Autodesk Inventor part; units mm, degrees
ref_plane "YZ Plane" through (0, 0, 0) normal (1, 0, 0) x (0, 1, 0)
ref_plane "XZ Plane" through (0, 0, 0) normal (0, 1, 0) x (-1, 0, 0)
ref_plane "XY Plane" through (0, 0, 0) normal (0, 0, 1) x (1, 0, 0)
sketch "Sketch1" plane through (0, 0, 0) normal (0, 0, 1) x (1, 0, 0)
  line L0 (0, 20.7) -> (0, 15)
  line L1 (29, 15) -> (95, 15)
  line L2 (95, 15) -> (95, 0)
  line L3 (95, 0) -> (-0.5001, 0)
  line L4 (-10.0501, 0) -> (123.65, 0)
  line L5 (-0.5001, 0) -> (-0.5001, 20.7)
  line L6 (-0.5001, 20.7) -> (0, 20.7)
  line L7 (29, 15) -> (26.8528, 15)
  line L8 (26.8528, 15) -> (0, 15)
  line L9 (0, -2.07) -> (0, 26.91)
  dimension "d0" = 95
  dimension "d1" = 66
  dimension "d2" = 30
  dimension "d9" = 0.5001
  dimension "d10" = 41.4
  dimension "d13" = 2.1472
  dimension "d14" = 30
revolve "Body" add sketch "Sketch1" angle 360 about axis through (95, 0, 0) along (-1, 0, 0)
sketch "Sketch2" plane through (-0.5001, 0, 0) normal (-1, 0, 0) x (0, 0, 1)
  line L0 (0, 26.5581) -> (23, 13.2791)
  line L1 (23, 13.2791) -> (23, -13.2791)
  line L2 (23, -13.2791) -> (0, -26.5581)
  line L3 (0, -26.5581) -> (-23, -13.2791)
  line L4 (-23, -13.2791) -> (-23, 13.2791)
  line L5 (-23, 13.2791) -> (0, 26.5581)
  point P0 (0, 0)
  point P1 (0, 0)
  dimension "d11" = 46
extrude "Head" add sketch "Sketch2" along normal blind 18.76
sketch "Sketch4" plane through (0, 0, 0) normal (0, 0, 1) x (1, 0, 0)
  line L0 (-19.2601, 23) -> (-19.2601, 26.5581)
  line L1 (-19.2601, 26.5581) -> (-17.2058, 26.5581)
  line L2 (-17.2058, 26.5581) -> (-19.2601, 23)
  line L3 (-21.1361, 0) -> (5.1279, 0)
  line L4 (-0.5001, 26.5581) -> (-19.2601, 26.5581)
  line L5 (-19.2601, 13.2791) -> (-19.2601, 26.5581)
  dimension "d5" = 30
  dimension "d19" = 46
revolve "Chamfer1" cut sketch "Sketch4" angle 360 about axis through (-10, 0, 0) along (1, 0, 0)
thread "Thread"
chamfer "Chamfer2" distance 2.1471 distance2 2.1472 1 edges at (95, -15, 0) measured on face at (95, -3.9999, 1.1966)
equation "\"d0\" = NLG"
equation "\"d1\" = GEL"
equation "\"d2\" = GD"
equation "\"d10\" = SD2"
equation "\"d14\" = BDM"
equation "\"d11\" = SW"
equation "\"d3\" = KOH - SD"
equation "\"d5\" = ANG1"
equation "\"d19\" = SW0"
equation "\"d15\" = GEL"
equation "\"d6\" = -0.5 * SPD + 0.5 * GD"
equation "\"NLG\" = 95"
equation "\"GD\" = NND"
equation "\"BDM\" = NND"
equation "\"KOH\" = 19.26"
equation "\"GEL\" = 66"
equation "\"SW\" = 46"
equation "\"SW0\" = 46"
equation "\"SPD\" = NND - 1.2269 * TPU"
equation "\"SD2\" = 0.9 * SW"
equation "\"SD\" = 0.5"
equation "\"ANG1\" = 30deg"
equation "\"GAL\" = 0.61345 * TPU"
equation "\"GUL\" = 0.61345 * TPU"
equation "\"RR\" = 1.7"
equation "\"d20\" = -NLG"
equation "\"TOA\" = 30deg"
equation "\"PTC\" = TPU"
equation "\"GD1\" = THREADDIA - 1.2269 * TPU"
equation "\"TPU\" = 3.5"
equation "\"E0\" = 1.155 * SW"
equation "\"SDH\" = 44.98"
properties part number "BS 3692 - M30 x 90"
Could you check a few things on this model? Use its own coordinates, in mm. A direction names the side the tool comes from. Round coordinates to 2 decimals unless told otherwise and drop trailing zeros. Loops run counter-clockwise (first coordinate to the right, second up) from the corner with the lowest first, then second, coordinate; pieces in that order, holes last. Notation, with made-up numbers: M 55,60 L 105,60 A14 ccw 105,82 Z; hole C 83,57 d1. An arc over 180 degrees is marked long. Answer as CSV lines item,"result".
1) For pin 1 Ø5 at (x, y) = (38.5, -4.5) entering from -Z; pin 2 Ø4 at (y, z) = (16.5, 16) entering from +X; pin 3 Ø5 at (x, y) = (7.5, -3) entering from -Z, each with a flat end and sliding along its axis, tell me the tip position at first contact or that it passes through.
From the geometry:
pin 1,"z = -14.87"
pin 2,"x = -0.5"
pin 3,"z = -14.99"
2) Which directions (+Z, -Z, +X, -X, +Y, -Y) give clear straight access to the entire face, cutting with the end or side of a thin tool? Please do faces 1 (the flat face through (-9.749, -19.826, 11.661)), 2 (the cylindrical face through (47.076, -14.985, 0.66)).
From the geometry:
face 1,"+Z, +X, -X, -Y"
face 2,"+X"
3) If I drill on probe 1 along X at (y, z) = (17.5, 14); probe 2 along X at (y, z) = (-15, 9); probe 3 along Y at (x, z) = (18.5, -0.5), over which ranges is the centre line in solid material (lowest first)?
From the geometry:
probe 1,"-19.26 to -0.5"
probe 2,"-19.26 to 0"
probe 3,"-14.99 to 14.99"
4) Imagine slicing it at A-A on x = 80. List the corners of the cut face in (y, z) for me.
From the geometry:
outline,"C 0,0 d30"
